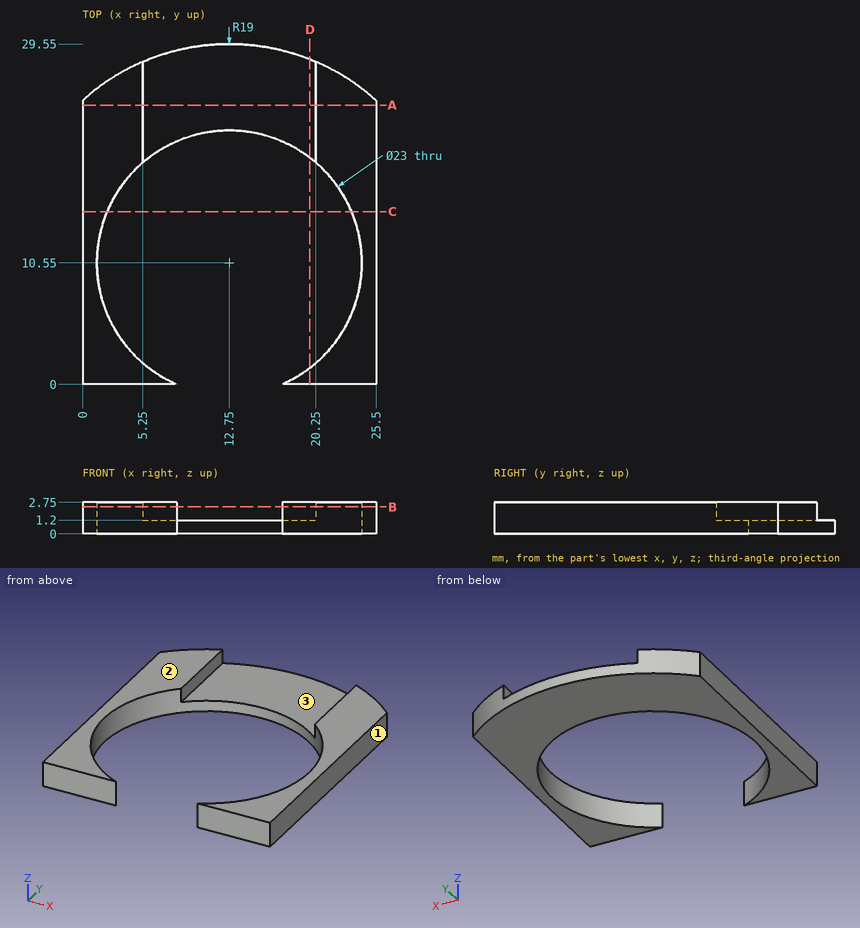
Here's the drawing with two shaded views (mm, measured from the low corner). I have some questions. Give positions to 0.01 mm unless a question says otherwise; leave off trailing zeros. Order: outer loops, then holes, each group sorted by start corner. A loop starts at its lowest first (then second) coordinate and runs counter-clockwise, first axis right, second up. Notation, with made-up numbers: (87.25, 17) - (106.25, 17) arc R25 ccw to (106.25, 32) - close; hole circle Ø10 at (-10.75, -29.5). An arc over 180 degrees is marked (long way). Use a Markdown table: item, result. Add a question column.
Q1. If we mould it in two halves opening along X, with no side actions, what happens to the marked faces 1, 2 and 3? For each: released by +X, released by -X, zero draft, split by the parting line, or undercut.
Q2. If we section it at B-B on z = 2.35: Write out the boundary of the cut face in (x, y), plus the area to 3 significant figures.
Q3. Please list where these lines run through material, in increasing order: line 1 along Z through (x, y) = (12, 23); line 2 along X through (y, z) = (14, 0.5); line 3 along X through (y, z) = (10.55, 0.6).
Q4. If we section it at A-A on y = 24.25: Write out the boundary of the cut face in (x, z).
Q5. If we section it at C-C on y = 15: Write out the boundary of the cut face in (x, z).
Q6. If we section it at D-D on x = 19.75: Write out the boundary of the cut face in (y, z).
Q7. I'm going to push flat-ended pins straight in: pin 1 (1 mm diameter, centred on x = 6.5, z = 2, fed in from +Y); pin 2 (5 mm diameter, centred on x = 12, y = 26, fed in from +Z). Where does each tip first touch, or does it pass through?
Answers follow:
| question | item | result |
|---|---|---|
| 1 | face 1 | released by +X |
| 1 | face 2 | zero draft |
| 1 | face 3 | undercut |
| 2 | outline | (0, 0) - (8.17, 0) arc R11.5 cw to (5.25, 19.27) - (5.25, 28.01) arc R19 ccw to (0, 24.64) - close; (17.33, 0) - (25.5, 0) - (25.5, 24.64) arc R19 ccw to (20.25, 28.01) - (20.25, 19.27) arc R11.5 cw to start |
| 2 | area | 186 mm^2 |
| 3 | line 1 | z = 0 to 1.2 |
| 3 | line 2 | x = 0 to 1.78, 23.72 to 25.5 |
| 3 | line 3 | x = 0 to 1.25, 24.25 to 25.5 |
| 4 | outline | (0, 0) - (25.5, 0) - (25.5, 2.75) - (20.25, 2.75) - (20.25, 1.2) - (5.25, 1.2) - (5.25, 2.75) - (0, 2.75) - close |
| 5 | outline | (0, 0) - (2.15, 0) - (2.15, 2.75) - (0, 2.75) - close; (23.35, 0) - (25.5, 0) - (25.5, 2.75) - (23.35, 2.75) - close |
| 6 | outline | (0, 0) - (1.43, 0) - (1.43, 2.75) - (0, 2.75) - close; (19.67, 0) - (28.21, 0) - (28.21, 1.2) - (19.67, 1.2) - close |
| 7 | pin 1 | stops at y = 1.24 |
| 7 | pin 2 | stops at z = 1.2 |
